Could you check a few things on this model? Use its own coordinates, in mm. Face numbers are marked on the shaded views. A direction names the side the tool comes from. Coordinates: 2 decimals unless noted, no trailing zeros. Order: outer loops, then holes, each group sorted by start corner. A loop starts at its lowest first (then second) coordinate and runs counter-clockwise, first axis right, second up. Notation, with made-up numbers: (77, -8) - (136, -8) arc R18 ccw to (136, 21) - close; hole circle Ø2 at (16, 29). An arc over 180 degrees is marked (long way). Answer as CSV lines item,"result". Start each with the question number.
1. For the marked faces 1, 2 and 3, which set-ups out of +Z, -Z, +X, -X, +Y, -Y let a thin tool reach every point of the face, with its end or its side?
2. I want a section at C-C, the plane x = 295.5. List the corners of the cut face in (y, z) for me, and give its area (3 significant figures).
3. I want a section at D-D, the plane x = -187. List the corners of the cut face in (y, z) for me.
4. I need wall thicknesses on probe 1 along Z at (x, y) = (33, 407); probe 2 along X at (y, z) = (92, 637.5); probe 3 along X at (y, z) = (128.5, 959.5). Which ranges of each line are inside material? Lowest first, please.
5. I want a section at B-B, the plane z = 286. List the corners of the cut face in (x, y) for me, and give its area (3 significant figures).
6. I want a section at A-A, the plane y = 313.5. List the corners of the cut face in (x, z) for me.
7. For pin 1 (10 mm diameter, centred on x = -265, y = 573, fed in from +Z); pin 2 (5 mm diameter, centred on y = 682.5, z = 501.5, fed in from +X); pin 3 (12 mm diameter, centred on y = 395, z = 221, fed in from +X), each with a flat end and sliding along its axis, tell me the tip position at first contact or that it passes through.
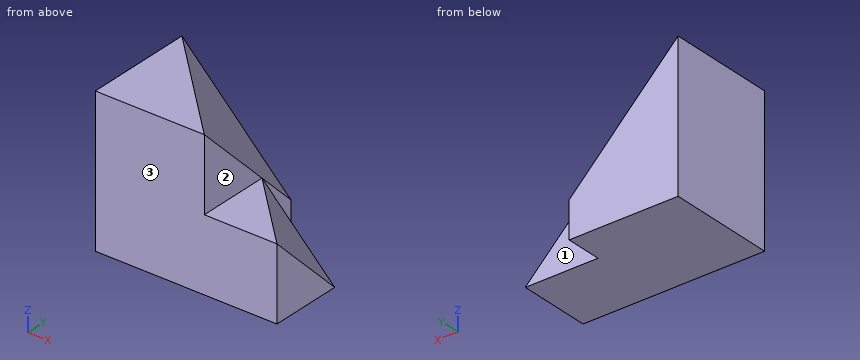
from build123d import *

# Parameters (mm, degrees)
SKETCH1_W           = 762
SKETCH1_H           = 762
BOSS_EXTRUDE2_DEPTH = 1016
SKETCH1_4_W         = 508
SKETCH1_4_H         = 508
BOSS_EXTRUDE3_DEPTH = 508


with BuildPart() as part:
    # Sketch1 → Boss-Extrude2 (new body)
    with BuildSketch(Plane.XY):
        with Locations((-381, 381)):
            Rectangle(SKETCH1_W, SKETCH1_H)
    extrude(amount=BOSS_EXTRUDE2_DEPTH)

    # Sketch1<4> → Boss-Extrude3 (add)
    with BuildSketch(Plane.XY):
        with Locations((254, 254)):
            Rectangle(SKETCH1_4_W, SKETCH1_4_H)
    extrude(amount=BOSS_EXTRUDE3_DEPTH)

    # SurfaceCut1
    split(bisect_by=Plane(origin=(338.666666667, 338.666666667, 338.666666667), x_dir=(0.816496580927726, -0.408248290463863, -0.408248290463863), z_dir=(0.5773502691896258, 0.5773502691896262, 0.5773502691896255)), keep=Keep.BOTTOM)


solid = part.part
Solved:
1,face 1,"+Z, -Z, +X, +Y"
1,face 2,"+Z, +X, +Y, -Y"
1,face 3,"+Z, -Z, +X, -X, -Y"
2,outline,"(0, 0) - (508, 0) - (508, 212.5) - (212.5, 508) - (0, 508) - close"
2,area,"214,000 mm2"
3,outline,"(0, 0) - (762, 0) - (762, 441) - (187, 1016) - (0, 1016) - close"
4,probe 1,"z = 0 to 508"
4,probe 2,"x = -762 to 0"
4,probe 3,"x = -762 to -72"
5,outline,"(-762, 0) - (508, 0) - (508, 222) - (222, 508) - (0, 508) - (0, 730) - (-32, 762) - (-762, 762) - close"
5,area,"797,000 mm2"
6,outline,"(-762, 0) - (508, 0) - (508, 194.5) - (194.5, 508) - (0, 508) - (0, 702.5) - (-313.5, 1016) - (-762, 1016) - close"
7,pin 1,"stops at z = 715.07"
7,pin 2,"stops at x = -164.46"
7,pin 3,"stops at x = 408.49"
